from build123d import *

# Parameters (mm, degrees)
SKETCH1_R            = 1.5
BOSS_EXTRUDE1_DEPTH  = 5
FILLET1_R            = 2
FILLET1_OF_MIRROR1_R = 2
FILLET2_R            = 2


with BuildPart() as part:
    # Sketch1 → Boss-Extrude1 (new body)
    with BuildSketch(Plane(origin=(0, 0, 0), x_dir=(1, 0, 0), z_dir=(0, 1, 0))):
        with BuildLine():
            Line((-58.655951842, -40), (-81.550499093, -23.96906543))
            ThreePointArc((-81.550499093, -23.96906543), (-84.423538078, 9.882622039), (-73.809947849, 42.155564266))
            Line((-73.809947849, 42.155564266), (-55.965512115, 60))
            Line((-55.965512115, 60), (-35, 60))
            Line((-35, 60), (-35, -27))
            Line((-35, -27), (0, -27))
            Line((0, -27), (0, -40))
            Line((0, -40), (-58.655951842, -40))
        make_face()
        with Locations((-43.840620434, 43.840620434)):
            Circle(SKETCH1_R, mode=Mode.SUBTRACT)
        with Locations((-51.997575213, -33.767620171)):
            Circle(SKETCH1_R, mode=Mode.SUBTRACT)
        with Locations((-59.39696962, 28.284271247)):
            Circle(SKETCH1_R, mode=Mode.SUBTRACT)
        with Locations((-79.5, 8.5)):
            Circle(SKETCH1_R, mode=Mode.SUBTRACT)
        Polygon((-65.5, 22.181240867), (-65.5, 20), (-70.5, 20), (-70.5, 15), (-65.5, 15), (-65.5, -15), (-70.5, -15), (-70.5, -20), (-65.5, -20), (-65.5, -23), (-56.256832596, -29.472135493), (-55, -23), (-51, -23), (-48.796166422, -28.387593469), (-40.5, -23), (-40.5, 30.600505063), (-44.547727215, 34.648232278), (-57.095959493, 22.1), (-59.095959493, 22.1), (-62.33860018, 25.342640687), align=None, mode=Mode.SUBTRACT)
    boss_extrude1 = extrude(amount=BOSS_EXTRUDE1_DEPTH)

    # Fillet1
    fillet1_edges = [part.edges().sort_by_distance(p)[0] for p in [
        (-44.547727215, 2.5, -34.648232278),
        (-62.33860018, 2.5, -25.342640687),
        (-56.256832596, 2.5, 29.472135493),
        (-48.796166422, 2.5, 28.387593469),
        (-40.5, 2.5, 23),
        (-40.5, 2.5, -30.600505063),
    ]]
    fillet(fillet1_edges, radius=FILLET1_R)

    # Mirror1: Boss-Extrude1 across plane
    add(boss_extrude1.mirror(Plane(origin=(0, 0, 0), x_dir=(0, 0, 1), z_dir=(1, 0, 0))))

    # Fillet1 of Mirror1
    fillet1_of_mirror1_edges = [part.edges().sort_by_distance(p)[0] for p in [
        (44.547727215, 2.5, -34.648232278),
        (62.33860018, 2.5, -25.342640687),
        (56.256832596, 2.5, 29.472135493),
        (48.796166422, 2.5, 28.387593469),
        (40.5, 2.5, 23),
        (40.5, 2.5, -30.600505063),
    ]]
    fillet(fillet1_of_mirror1_edges, radius=FILLET1_OF_MIRROR1_R)

    # Fillet2
    fillet2_edges = [part.edges().sort_by_distance(p)[0] for p in [
        (-55.965512115, 2.5, -60),
        (-35, 2.5, -60),
        (-58.655951842, 2.5, 40),
        (55.965512115, 2.5, -60),
        (35, 2.5, -60),
        (58.655951842, 2.5, 40),
    ]]
    fillet(fillet2_edges, radius=FILLET2_R)


solid = part.part
Verification items for the finished model (mm, model axes). A direction names the side the tool comes from. Coordinates: 2 decimals unless noted, no trailing zeros. Order: outer loops, then holes, each group sorted by start corner. A loop starts at its lowest first (then second) coordinate and runs counter-clockwise, first axis right, second up. Notation, with made-up numbers: M 75,17.25 L 119,17.25 A16 ccw 119,36.25 Z; hole C -2,59 d1. An arc over 180 degrees is marked long. Return JSON: item names as keys, results as strings.
1) Thickness scan on L1, parallel to Z at x = 66, y = 1.65; L2, parallel to X at y = 1.2, z = 3.5; L3, parallel to Z at x = 68.5, y = 2.95. Record the ranges inside material, lowest first. Write a range as [from, to].
Answer list:
{"L1": "[-49.97, -20], [-15, 15], [20, 34.86]", "L2": "[-84.93, -65.5], [-40.5, -35], [35, 40.5], [65.5, 84.93]", "L3": "[-47.47, -20], [-15, 15], [20, 33.11]"}
2) Cross-section at D-D, the plane y = 4.2. Count the separate pieces of the cut face and the enclosed holes in it, and give its area (3 significant figures).
Answer list:
{"separate pieces": "1", "enclosed holes": "10", "area": "6,560 mm2"}
3) Cross-section at A-A, the plane z = -36.5. Record the boundary of the cut face in (x, y), and give its area (3 significant figures).
Answer list:
{"outline": "M -76.76,0 L -35,0 L -35,5 L -76.76,5 Z; M 35,0 L 76.76,0 L 76.76,5 L 35,5 Z", "area": "418 mm2"}
4) Cross-section at C-C, the plane x = 20.5. Record the boundary of the cut face in (y, z).
Answer list:
{"outline": "M 0,27 L 5,27 L 5,40 L 0,40 Z"}
5) Gauge pin test, flat ends, axial feed: pin 1 (2.5 mm diameter, centred on y = 2, z = -14, fed in from +X); pin 2 (2.5 mm diameter, centred on x = -67, y = 2.5, fed in from +Z); pin 3 (3 mm diameter, centred on y = 2, z = 29.5, fed in from -X). Record the tip position at first contact, or that the pin passes through.
Answer list:
{"pin 1": "x = 84.04", "pin 2": "z = 35.03", "pin 3": "x = -75.79"}
6) Cross-section at B-B, the plane z = -17. Record the boundary of the cut face in (x, y).
Answer list:
{"outline": "M -83.28,0 L -70.5,0 L -70.5,5 L -83.28,5 Z; M -40.5,0 L -35,0 L -35,5 L -40.5,5 Z; M 35,0 L 40.5,0 L 40.5,5 L 35,5 Z; M 70.5,0 L 83.28,0 L 83.28,5 L 70.5,5 Z"}
7) Release check for a two-part mould opening along Z. For faces 1 (the flat face through (46, 2, -60)), 2 (the cylindrical face through (-58.705, 2.465, -26.954)), 3 (the cylindrical face through (84.478, 2.465, -9.407)) record: +Z half, -Z half, draft (parallel to the pull), parting line (faces both ways), or undercut.
Answer list:
{"face 1": "-Z half", "face 2": "undercut", "face 3": "parting line"}
8) Access from +Z, -Z, +X, -X, +Y, -Y to the whole of each face (thin tool, end or side, straight path). Record for faces 4 (the flat face through (-51.451, 2.465, -27.745)), 5 (the flat face through (-1, 2, 40)).
Answer list:
{"face 4": "+Y, -Y", "face 5": "+Z, +X, -X, +Y, -Y"}
